The figure shows three views and two pictorial views of one solid part (mm, origin at its lowest corner). Answer the questions. A direction names the side the tool comes from. Coordinates: 2 decimals unless noted, no trailing zeros. Loops run counter-clockwise (first coordinate to the right, second up) from the corner with the lowest first, then second, coordinate; pieces in that order, holes last. Notation, with made-up numbers: (-5, 16) -> (38, 16) arc R22 cw to (38, 45) -> close; hole circle Ø2 at (13, 82.5). An arc over 180 degrees is marked (long way). Answer as a JSON object with one key per item and string values. Group by question number.
1) Flat-ended cylindrical pins translate along their axes: P1, Ø6.5, axis at x = 20, z = 10, coming from the +Y side; P2, Ø4, axis at x = 165, y = 32.5, coming from the +Z side; P3, Ø3, axis at y = 53.5, z = 72.5, coming from the -X side. Find the tip coordinate at first contact, or state that the pin passes through.
2) Which of the six approach directions +Z, -Z, +X, -X, +Y, -Y give full straight-line access (tool end or side, diameter ignored) to the marked faces 1, 2 and 3?
3) Section A-A, the plane x = 230 is taken. Give the vertices of the cut face in (y, z).
4) Section C-C, the plane x = 64 is taken. Give the vertices of the cut face in (y, z).
5) Section B-B, the plane z = 47 is taken. Give the vertices of the cut face in (x, y), plus the area to 3 significant figures.
6) Consider probe 1 along X at (y, z) = (6.25, 10); probe 2 along Z at (x, y) = (230, 4); probe 3 along Z at (x, y) = (157.5, 55.5). Determine where each line is inside the solid, lowest interval first. Write a range as [from, to].
7) Section D-D, the plane y = 30 is taken. Give the vertices of the cut face in (x, z), plus the area to 3 significant figures.
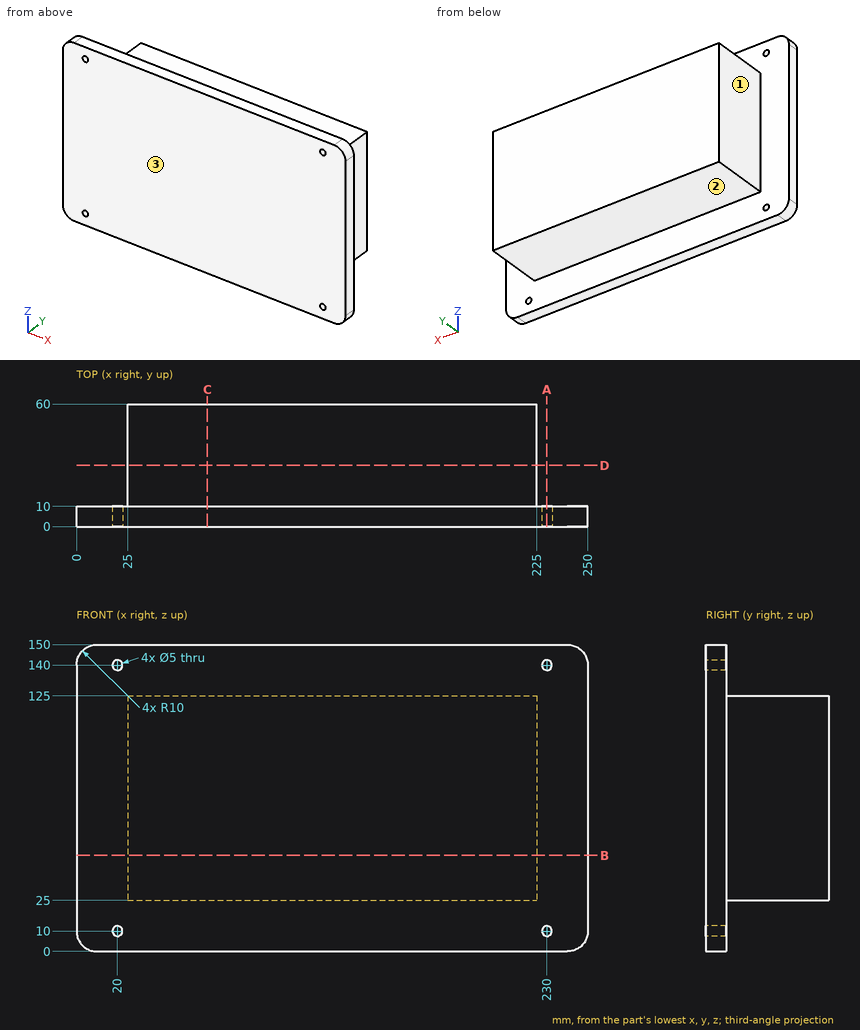
Determined:
{
 "1": {"P1": "y = 10", "P2": "z = 125", "P3": "x = 25"},
 "2": {"face 1": "+Z, -Z, -X, +Y", "face 2": "-Z, +X, -X, +Y", "face 3": "+Z, -Z, +X, -X, -Y"},
 "3": {"outline": "(0, 0) -> (10, 0) -> (10, 7.5) -> (0, 7.5) -> close; (0, 12.5) -> (10, 12.5) -> (10, 137.5) -> (0, 137.5) -> close; (0, 142.5) -> (10, 142.5) -> (10, 150) -> (0, 150) -> close"},
 "4": {"outline": "(0, 0) -> (10, 0) -> (10, 25) -> (60, 25) -> (60, 125) -> (10, 125) -> (10, 150) -> (0, 150) -> close"},
 "5": {"outline": "(0, 0) -> (250, 0) -> (250, 10) -> (225, 10) -> (225, 60) -> (25, 60) -> (25, 10) -> (0, 10) -> close", "area": "12,500 mm²"},
 "6": {"probe 1": "[0, 17.5], [22.5, 227.5], [232.5, 250]", "probe 2": "[0, 7.5], [12.5, 137.5], [142.5, 150]", "probe 3": "[25, 125]"},
 "7": {"outline": "(25, 25) -> (225, 25) -> (225, 125) -> (25, 125) -> close", "area": "20,000 mm²"}
}
